Could you check a few things on this model? Use its own coordinates, in mm. Round coordinates to 2 decimals unless told otherwise and drop trailing zeros. Loops run counter-clockwise (first coordinate to the right, second up) from the corner with the lowest first, then second, coordinate; pieces in that order, holes last. Notation, with made-up numbers: (-28.75, -1) -> (28.25, -1) arc R19 ccw to (28.25, 24) -> close; hole circle Ø7 at (41.5, 58.5). An arc over 180 degrees is marked (long way). One line per item, written item: value.
```python
from build123d import *

# Parameters (mm, degrees)
SKETCH1_W           = 140
SKETCH1_H           = 100
BOSS_EXTRUDE1_DEPTH = 100
SKETCH2_R           = 41
CUT_EXTRUDE1_DEPTH  = 163.215905518
SKETCH3_W           = 20
SKETCH3_H           = 100
CUT_EXTRUDE2_DEPTH  = 101
SKETCH4_W           = 10
SKETCH4_H           = 100
CUT_EXTRUDE3_DEPTH  = 101
SKETCH5_R           = 41
BOSS_EXTRUDE2_DEPTH = 20.3
CUT_EXTRUDE4_DEPTH  = 101


with BuildPart() as part:
    # Sketch1 → Boss-Extrude1 (new body)
    with BuildSketch(Plane.XY):
        Rectangle(SKETCH1_W, SKETCH1_H)
    extrude(amount=BOSS_EXTRUDE1_DEPTH)

    # Sketch2 → Cut-Extrude1 (cut, through all)
    with BuildSketch(Plane(origin=(-70.013926023, 0, 99.990248894), x_dir=(0, -1, 0), z_dir=(-0.573576436, 0, 0.819152044))):
        with Locations((0, 58.017000535)):
            Circle(SKETCH2_R)
    extrude(amount=-CUT_EXTRUDE1_DEPTH, mode=Mode.SUBTRACT)

    # Sketch3 → Cut-Extrude2 (cut, through all)
    with BuildSketch(Plane.XY.offset(100)):
        with Locations((-60, 0)):
            Rectangle(SKETCH3_W, SKETCH3_H)
    extrude(amount=-CUT_EXTRUDE2_DEPTH, mode=Mode.SUBTRACT)

    # Sketch4 → Cut-Extrude3 (cut, through all)
    with BuildSketch(Plane.XY.offset(100)):
        with Locations((-45, 0)):
            Rectangle(SKETCH4_W, SKETCH4_H)
        with Locations((65, 0)):
            Rectangle(SKETCH4_W, SKETCH4_H)
    extrude(amount=-CUT_EXTRUDE3_DEPTH, mode=Mode.SUBTRACT)

    # Sketch5 → Boss-Extrude2 (add)
    with BuildSketch(Plane(origin=(19.7393957, 0, -28.190778624), x_dir=(-0.819152044, 0, -0.573576436), z_dir=(0.573576436, 0, -0.819152044))):
        with Locations((-58.017000535, 0)):
            Circle(SKETCH5_R)
    extrude(amount=-BOSS_EXTRUDE2_DEPTH)

    # Sketch6 → Cut-Extrude4 (cut, through all)
    with BuildSketch(Plane(origin=(0, 50, 0), x_dir=(1, 0, 0), z_dir=(0, 1, 0))):
        Polygon((60, 0), (-40, 0), (-40, 38.622200476), (122.468168518, 38.622200476), (119.926290674, -91.2591408), (60, -91.2591408), align=None)
    extrude(amount=-CUT_EXTRUDE4_DEPTH, mode=Mode.SUBTRACT)


solid = part.part
```
Item 1: If we section it at C-C on y = -7.5: List the corners of the cut face in (x, z) for me.
Output:
outline: (-40, 0) -> (21.62, 0) -> (-40, 88) -> close; (24.61, 0) -> (60, 0) -> (60, 24.78) -> close; (50.01, 100) -> (60, 85.74) -> (60, 100) -> close
Item 2: I need wall thicknesses on line 1 (Y direction, x = 20.5, z = 71); line 2 (Y direction, x = 19, z = 39); line 3 (X direction, y = 9.5, z = 12.5). Which ranges of each line are inside material? Lowest first, please. Write a range as from..to.
Output:
line 1: y = -50..-41, 41..50
line 2: y = -50..-35.74, 35.74..50
line 3: x = -40..13.38, 42.46..60
Item 3: If we section it at A-A on y = 29.5: List the corners of the cut face in (x, z) for me (3 decimals), plus the area to 3 significant figures.
Output:
outline: (-40, 0) -> (60, 0) -> (60, 24.782) -> (32.296, 5.383) -> (-33.955, 100) -> (-40, 100) -> close; (35.565, 100) -> (60, 65.103) -> (60, 100) -> close
area: 4,940 mm²
Item 4: Will these pins go through, and if not, where does the flat tip stop? pin 1 Ø12 at (x, y) = (-18.5, -11) entering from +Z; pin 2 Ø1 at (y, z) = (7, 27) entering from +X.
Output:
pin 1: stops at z = 67.87
pin 2: stops at x = 2.97
Item 5: If we section it at B-B on y = 4: List the corners of the cut face in (x, z) for me, plus the area to 3 significant figures.
Output:
outline: (-40, 0) -> (21.01, 0) -> (-40, 87.14) -> close; (24.61, 0) -> (60, 0) -> (60, 24.78) -> close; (50.62, 100) -> (60, 86.6) -> (60, 100) -> close
area: 3,160 mm²
Item 6: If we mould it in two halves opening along X, with no side actions, what happens to faces 1 (the face through (9, 50, 49)), 2 (the face through (60, -1, 17)), 3 (the face through (42.6, 0.6, 12.6))? For each: released by +X, released by -X, zero draft, split by the parting line, or undercut.
Output:
face 1: zero draft
face 2: released by +X
face 3: undercut
